from build123d import *

# Parameters (mm, degrees)
MODEL_R           = 1.4
MODEL_R_2         = 1
BRIDA_BASE1_DEPTH = 1


# Sheet-metal steps are written as plain solids
with BuildPart() as part:
    # Model → Brida base1 (new body)
    with BuildSketch(Plane.XY):
        with BuildLine():
            Line((60.2059904, 3.7384384), (50.2059904, 3.7384384))
            Line((50.2059904, 3.7384384), (50.2059904, -15.7615616))
            ThreePointArc((50.2059904, -15.7615616), (45.2059904, -20.7615616), (40.2059904, -15.7615616))
            Line((40.2059904, -15.7615616), (40.2059904, 3.7384384))
            Line((40.2059904, 3.7384384), (30.2059904, 3.7384384))
            ThreePointArc((30.2059904, 3.7384384), (23.46215545, 27.372628124), (2.911625265, 40.853352987))
            ThreePointArc((2.911625265, 40.853352987), (0.630018379, 43.781083427), (3.040300155, 46.603826289))
            ThreePointArc((3.040300155, 46.603826289), (40.977818177, 37.646613371), (60.2059904, 3.7384384))
        make_face()
        with Locations((45.2059904, -15.7615616)):
            Circle(MODEL_R, mode=Mode.SUBTRACT)
        with Locations((45.2059904, -3.2615616)):
            Circle(MODEL_R_2, mode=Mode.SUBTRACT)
    extrude(amount=-BRIDA_BASE1_DEPTH)


solid = part.part
Input: part model. Units: mm. Frame: model coordinates. Coordinates: 2 decimals unless noted, no trailing zeros. Order: outer loops, then holes, each group sorted by start corner. A loop starts at its lowest first (then second) coordinate and runs counter-clockwise, first axis right, second up. Notation, with made-up numbers: M 59,50.5 L 102,50.5 A33 ccw 102,80.5 Z; hole C 40.25,-25 d11. An arc over 180 degrees is marked long. Write item = value, one per line. Start each with the question number.
(1) Pull-direction query (Y, two-part tool) for faces 1 (the cylindrical face through (44.09, -16.61, -0.49)), 2 (the cylindrical face through (45.32, -20.76, -0.49)), 3 (the cylindrical face through (0.63, 43.72, -0.49)); classes: released by +Y, released by -Y, zero draft, split by the parting line, or undercut.
(2) Section C-C on y = -13.5. Output: boundary loops of the cut face in (x, z), and give its area (3 significant figures).
(3) Section B-B on z = -0.5. Output: boundary loops of the cut face in (x, y), and give its area (3 significant figures).
(4) Section D-D on x = 55. Output: boundary loops of the cut face in (y, z), and give its area (3 significant figures).
(5) First-contact query: P1, Ø0.5, axis at y = -10.5, z = -0.5, coming from the -X side. Flat tip, straight axial feed; report the tip coordinate or a pass-through.
(6) Section A-A on x = 45. Output: boundary loops of the cut face in (y, z).
(7) Line query: line 1 along Y through (x, z) = (45, -0.15); line 2 along X through (y, z) = (-12.5, -0.45); line 3 along X through (y, z) = (27.5, -0.1). Output: solid intervals per line, ascending. Write a range as [from, to].
Result set:
q1.face_1 = undercut
q1.face_2 = released by -Y
q1.face_3 = split by the parting line
q2.outline = M 40.21,-1 L 50.21,-1 L 50.21,0 L 40.21,0 Z
q2.area = 10.0 mm²
q3.outline = M 2.91,40.85 A35.25 cw 30.21,3.74 L 40.21,3.74 L 40.21,-15.76 A5 ccw 50.21,-15.76 L 50.21,3.74 L 60.21,3.74 A48.72 ccw 3.04,46.6 A2.94 ccw Z; hole C 45.21,-15.76 d2.8; hole C 45.21,-3.26 d2
q3.area = 1,460 mm²
q4.outline = M 3.74,-1 L 21.1,-1 L 21.1,0 L 3.74,0 Z
q4.area = 17.4 mm²
q5.P1 = 40.21
q6.outline = M -20.76,-1 L -17.15,-1 L -17.15,0 L -20.76,0 Z; M -14.38,-1 L -4.24,-1 L -4.24,0 L -14.38,0 Z; M -2.28,-1 L 34.28,-1 L 34.28,0 L -2.28,0 Z
q7.line_1 = [-20.76, -17.15], [-14.38, -4.24], [-2.28, 34.28]
q7.line_2 = [40.21, 50.21]
q7.line_3 = [23.37, 51.02]
